Input: dimensioned drawing with shaded views. Units: mm. Origin: part minimum x, y, z. Coordinates: 2 decimals unless noted, no trailing zeros. Write each loop counter-clockwise with the first axis right and the second up, starting at its lowest first coordinate (ties: lowest second). Pieces come first, ordered by that corner, then holes. Notation, with made-up numbers: (-21, 75.25) - (3, 75.25) arc R23 ccw to (3, 95.25) - close; hole circle Ø5 at (-17.5, -36.75). An arc over 180 degrees is marked (long way). One line per question, with ' | ' between items.
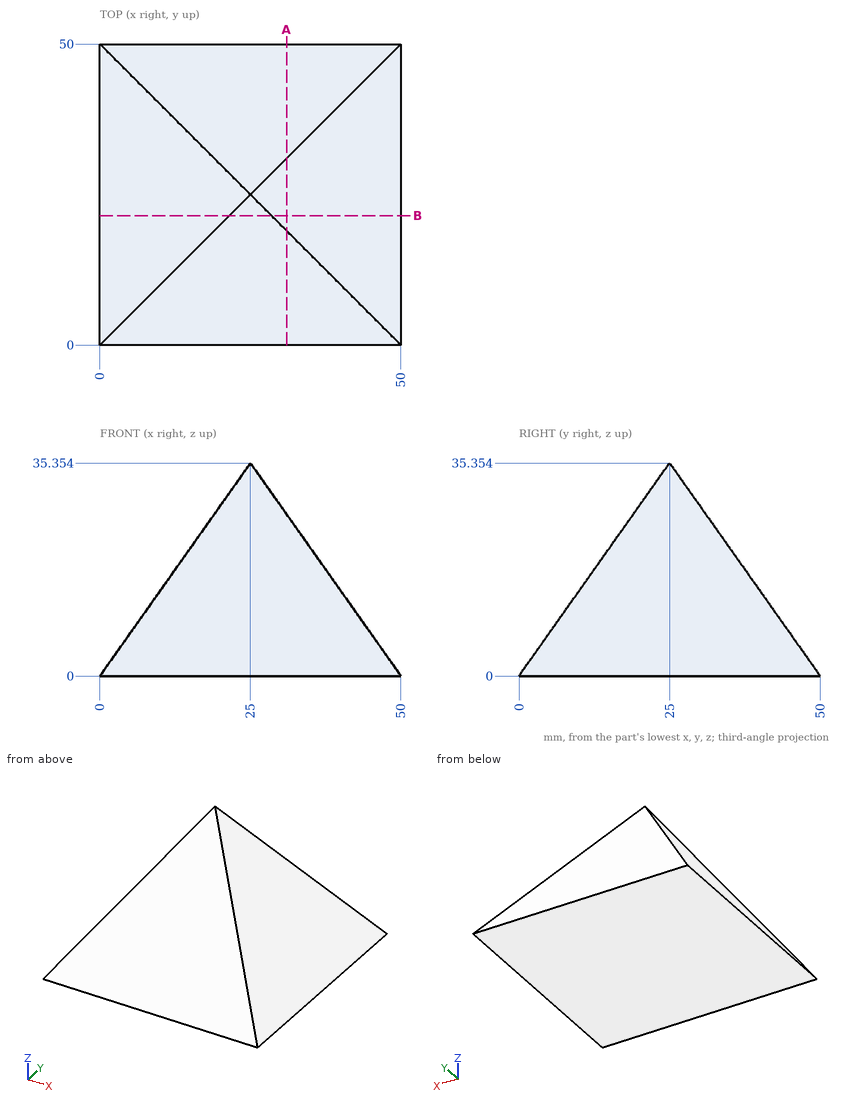
Item 1: Ray query, line 1 along Y through (x, z) = (41.5, 3.5) (1 decimal); line 2 along X through (y, z) = (33, 10.5) (1 decimal); line 3 along Y through (x, z) = (20, 6). Return the intervals inside material, ascending. Write a range as [from, to].
Check sheet entries:
line 1: [2.5, 47.5] | line 2: [7.4, 42.6] | line 3: [4.24, 45.76]
Item 2: Cut plane A-A on x = 31. Return loops of the section in (y, z).
Check sheet entries:
outline: (0, 0) - (50, 0) - (31, 26.87) - (19, 26.87) - close
Item 3: Cut plane B-B on y = 21.5. Return loops of the section in (x, z).
Check sheet entries:
outline: (0, 0) - (50, 0) - (28.5, 30.4) - (21.5, 30.4) - close
Item 4: Pin query (flat end, axial travel): pin 1 Ø6 at (x, z) = (34, 26.5) entering from +Y; pin 2 Ø4 at (x, z) = (8.5, 17.5) entering from -Y; pin 3 Ø3 at (x, y) = (43, 15.5) entering from +Z; pin 4 Ø10 at (x, y) = (24.5, 12) entering from +Z. Return the tip coordinate at first contact, or that it passes through.
Check sheet entries:
pin 1: y = 33.33 | pin 2: through | pin 3: z = 12.02 | pin 4: z = 24.04
